Part model, mm, in its own coordinate system. A direction names the side the tool comes from. Give positions to 0.01 mm unless a question says otherwise; leave off trailing zeros. Loops run counter-clockwise (first coordinate to the right, second up) from the corner with the lowest first, then second, coordinate; pieces in that order, holes last. Notation, with made-up numbers: (45, -17) -> (57, -17) arc R12 cw to (57, -1) -> close; hole circle Ø3 at (-21.5, 86). An arc over 180 degrees is marked (long way). Write item = value, one per line.
from build123d import *

# Parameters (mm, degrees)
PAD012_DEPTH    = 10
SKETCH061_W     = 3.35
SKETCH061_H     = 5.5
POCKET011_DEPTH = 5.7141437505


with BuildPart() as part:
    # Sketch059 → Pad012 (new body, symmetric)
    with BuildSketch(Plane.YZ):
        with BuildLine():
            ThreePointArc((-21.8787366497, 7.7856764323), (-24.5162755283, 6.5038208287), (-26.9380130719, 4.8500516808))
            ThreePointArc((-26.9380130719, 4.8500516808), (-27.1193333278, 4.5434596832), (-27.0505550432, 4.1939668567))
            Line((-27.0505550432, 4.1939668567), (-26.6017940465, 3.4757991384))
            ThreePointArc((-26.6017940465, 3.4757991384), (-25.5113742234, 2.6980102375), (-24.1903511659, 2.9190736826))
            Line((-24.1903511659, 2.9190736826), (-20.840561186, 5.0122547763))
            ThreePointArc((-20.840561186, 5.0122547763), (-20.3961103855, 5.6353518181), (-20.5224323541, 6.3902221367))
            Line((-21.2697124354, 7.5861202536), (-20.5224323541, 6.3902221367))
            ThreePointArc((-21.2697124354, 7.5861202536), (-21.5380484263, 7.7963039987), (-21.8787366497, 7.7856764323))
        make_face()
    extrude(amount=PAD012_DEPTH, both=True)

    # Sketch061 (on Face6 of Pad012) → Pocket011 (cut, through all)
    with BuildSketch(Plane(origin=(0, -8.1048226153, 12.9704274831), x_dir=(0, 0.8480480962, 0.5299192642), z_dir=(0, 0.5299192642, -0.8480480962))):
        with Locations((-19.0427078734, 7.25)):
            Rectangle(SKETCH061_W, SKETCH061_H)
        with Locations((-19.0427078734, -7.25)):
            Rectangle(SKETCH061_W, SKETCH061_H)
    extrude(amount=-POCKET011_DEPTH, mode=Mode.SUBTRACT)

    # SubtractivePipe002: sweep along a path in Sketch063
    with BuildLine(Plane.YZ.offset(4.5)) as subtractivepipe002_path:
        ThreePointArc((-21.4885664226, 7.9363598462), (-24.5285349663, 6.4967015301), (-27.284244153, 4.5679476082))
    # Sketch062 (on DatumPlane) → SubtractivePipe002 (sweep, cut)
    with BuildSketch(Plane(origin=(4.5, -26.9380130719, 4.8500516808), x_dir=(0, -0.6229641536, 0.782250384), z_dir=(0, -0.782250384, -0.6229641536))):
        Polygon((0, -0.025), (0, 0.025), (-0.0433012702, 0), align=None)
    subtractivepipe002 = sweep(path=subtractivepipe002_path.line, mode=Mode.SUBTRACT)

    # Mirrored002: SubtractivePipe002 across YZ
    add(subtractivepipe002.mirror(Plane.YZ), mode=Mode.SUBTRACT)


solid = part.part
1) Slice it at B-B, the plane z = 3.25. List the corners of the cut face in (x, y).
Resolved:
outline = (-4.5, -26.43) -> (4.5, -26.43) -> (4.5, -23.66) -> (-4.5, -23.66) -> close
2) Which spindle directions (+Z, -Z, +X, -X, +Y, -Y) get a long thin tool onto all of the face, cutting with end or side? Do faces 1 (the face through (10, -22, 6)), 2 (the face through (7.212, -23.673, 5.11)), 3 (the face through (-7.288, -23.673, 5.11)). Say none if no direction does.
Resolved:
face_1 = +Z, -Z, +X, +Y, -Y
face_2 = -Z, +X, -Y
face_3 = -Z, -X, -Y
3) Slice it at A-A, the plane x = 2. List the corners of the cut face in (y, z), and give its area (3 significant figures).
Resolved:
outline = (-27.05, 4.19) -> (-26.6, 3.48) arc R1.75 ccw to (-24.19, 2.92) -> (-20.84, 5.01) arc R1 ccw to (-20.52, 6.39) -> (-21.27, 7.59) arc R0.5 ccw to (-21.88, 7.79) arc R20 ccw to (-26.94, 4.85) arc R0.5 ccw to start
area = 20.0 mm²
4) Drop flat-ended pins along their axis: P1, Ø1.5, axis at x = -3, z = 7, coming from the +Y side; P2, Ø3, axis at y = -25.5, z = 4, coming from the +X side; P3, Ø1, axis at x = 0, z = 7, coming from the -Y side; P4, Ø3, axis at y = -24, z = 4, coming from the -X side. Give the stop position or say it passes through.
Resolved:
P1 = -20.45
P2 = 4.5
P3 = -24.52
P4 = -10
5) Drill centre lines: line 1 along X through (y, z) = (-25.75, 4.55); line 2 along Z through (x, y) = (1.75, -23.25); line 3 along Y through (x, z) = (0.5, 6.15). Where is each one in solid material? Low to high. Write a range as [from, to].
Resolved:
line_1 = [-4.5, 4.5]
line_2 = [3.51, 7.18]
line_3 = [-25.1, -20.41]
6) Slice it at C-C, the plane x = 5. List the corners of the cut face in (y, z).
Resolved:
outline = (-24.54, 6.49) -> (-22.83, 3.77) -> (-20.84, 5.01) arc R1 ccw to (-20.52, 6.39) -> (-21.27, 7.59) arc R0.5 ccw to (-21.88, 7.79) arc R20 ccw to start
